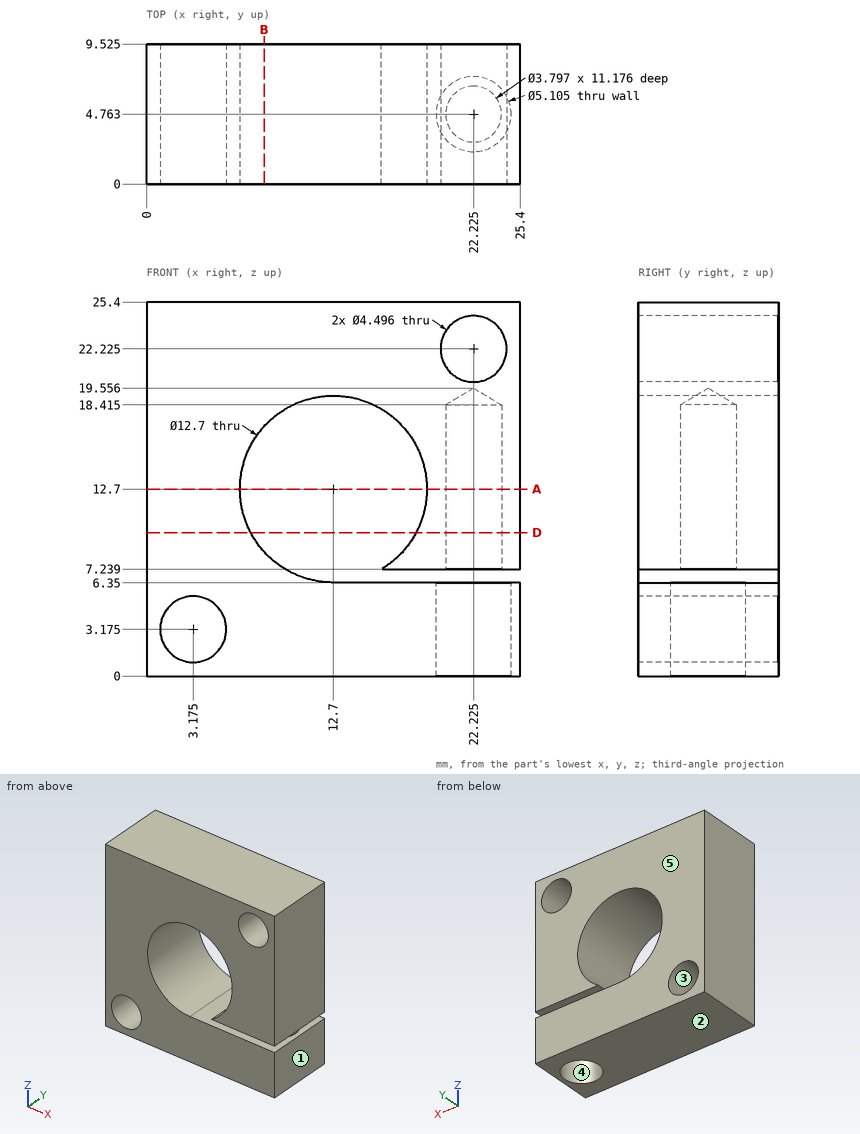
Geometry: see drawing. Coordinates: mm, zero at the bounding-box minimum. A direction names the side the tool comes from. Give positions to 0.01 mm unless a question says otherwise; leave off trailing zeros. Loops run counter-clockwise (first coordinate to the right, second up) from the corner with the lowest first, then second, coordinate; pieces in that order, holes last. Notation, with made-up numbers: (-3.5, 81) -> (15.5, 81) arc R18 ccw to (15.5, 115) -> close; hole circle Ø4 at (-36, -38). An arc over 180 degrees is marked (long way). Answer as a JSON object with one key per item and string values. Group by question number.
Item 1: Pull-direction query (Z, two-part tool) for the marked faces 1, 2 and 3; classes: released by +Z, released by -Z, zero draft, split by the parting line, or undercut.
Item 2: Cut plane B-B, the plane x = 8. Return the cut outline in (y, z) (1 decimal), and give its area (3 significant figures).
Item 3: Reachability of the marked faces 4 and 5 from +Z, -Z, +X, -X, +Y, -Y: full face, straight path, thin tool, end or side. Return the list, or none.
Item 4: Cut plane D-D, the plane z = 9.75. Return the cut outline in (x, y) (1 decimal).
Item 5: Line query: probe 1 along X at (y, z) = (4.75, 12.7); probe 2 along Z at (x, y) = (21.5, 8.75); probe 3 along Z at (x, y) = (21, 1.75). Output: solid intervals per line, ascending.
Item 6: Cut plane A-A, the plane z = 12.7. State how many separate pieces and enclosed holes the cut face has, and give its area (3 significant figures).
Checks:
{
 "1": {"face 1": "zero draft", "face 2": "released by -Z", "face 3": "undercut"},
 "2": {"outline": "(0, 0) -> (9.5, 0) -> (9.5, 8.4) -> (0, 8.4) -> close; (0, 17) -> (9.5, 17) -> (9.5, 25.4) -> (0, 25.4) -> close", "area": "161 mm²"},
 "3": {"face 4": "-Z", "face 5": "+Z, -Z, +X, -X, +Y"},
 "4": {"outline": "(0, 0) -> (7.1, 0) -> (7.1, 9.5) -> (0, 9.5) -> close; (18.3, 0) -> (25.4, 0) -> (25.4, 9.5) -> (18.3, 9.5) -> close; hole circle Ø3.8 at (22.2, 4.8)"},
 "5": {"probe 1": "x = 0 to 6.35, 19.05 to 20.33, 24.12 to 25.4", "probe 2": "z = 0 to 6.35, 7.24 to 20.1, 24.35 to 25.4", "probe 3": "z = 0 to 6.35, 7.24 to 20.34, 24.11 to 25.4"},
 "6": {"separate pieces": "2", "enclosed holes": "1", "area": "110 mm²"}
}
